Source: three-view drawing plus pictorial views. Frame: mm from the lowest corner of the part. Give positions to 0.01 mm unless a question says otherwise; leave off trailing zeros. Loops run counter-clockwise (first coordinate to the right, second up) from the corner with the lowest first, then second, coordinate; pieces in that order, holes last. Notation, with made-up numbers: (-21, 21) - (36, 21) arc R18 ccw to (36, 33) - close; hole circle Ø1 at (62.5, 44.5). An arc over 180 degrees is marked (long way). One line per item, written item: value.
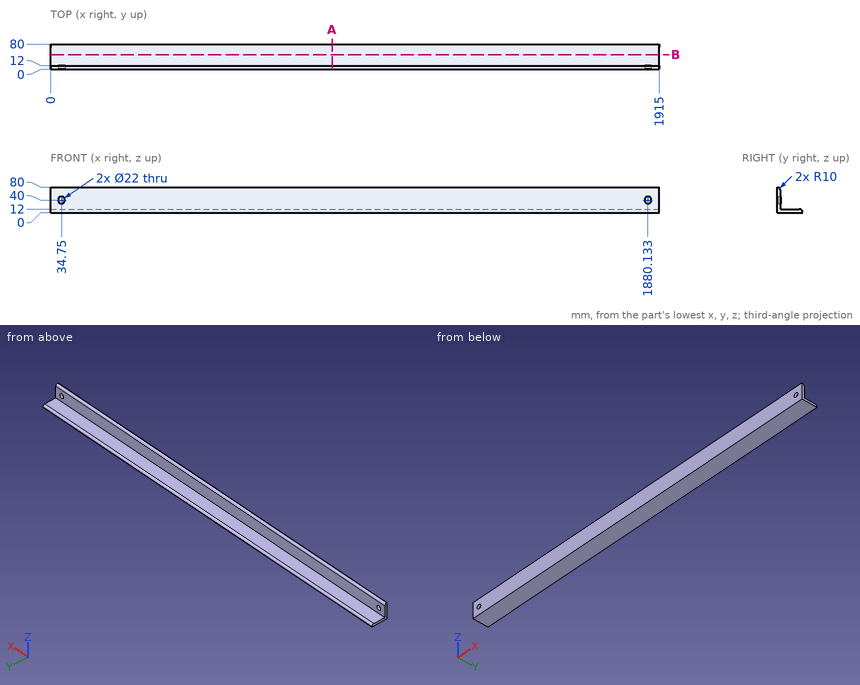
Item 1: Section B-B, the plane y = 46.5. Output: boundary loops of the cut face in (x, z).
Verdict:
outline: (0, 0) - (1915, 0) - (1915, 12) - (0, 12) - close
Item 2: Pin query (flat end, axial travel): P1, Ø1.5, axis at x = 1247, z = 41.5, coming from the +Y side; P2, Ø8, axis at x = 214, y = 45, coming from the -Z side. Return the tip coordinate at first contact, or that it passes through.
Verdict:
P1: stops at y = 12
P2: stops at z = 0
Item 3: Section A-A, the plane x = 886.5. Output: boundary loops of the cut face in (y, z).
Verdict:
outline: (0, 0) - (80, 0) - (80, 2) arc R10 ccw to (70, 12) - (12, 12) - (12, 70) arc R10 ccw to (2, 80) - (0, 80) - close
Item 4: Material intervals for L1, parallel to X at y = 6.5, z = 40; L2, parallel to Y at x = 1755, z = 3; L3, parallel to Z at x = 1263.5, y = 51, sorted ascending.
Verdict:
L1: x = 0 to 23.75, 45.75 to 1869.13, 1891.13 to 1915
L2: y = 0 to 79.95
L3: z = 0 to 12
